Geometry check sheet. Reference: the model listing, model coordinates, mm. Coordinates: 2 decimals unless noted, no trailing zeros. Order: outer loops, then holes, each group sorted by start corner. A loop starts at its lowest first (then second) coordinate and runs counter-clockwise, first axis right, second up. Notation, with made-up numbers: (36, 7) -> (65, 7) arc R29 cw to (65, 30) -> close; hole circle Ø5 at (26.5, 11). An arc over 180 degrees is marked (long way). Answer in a Markdown table with one row per item. Add a question column.
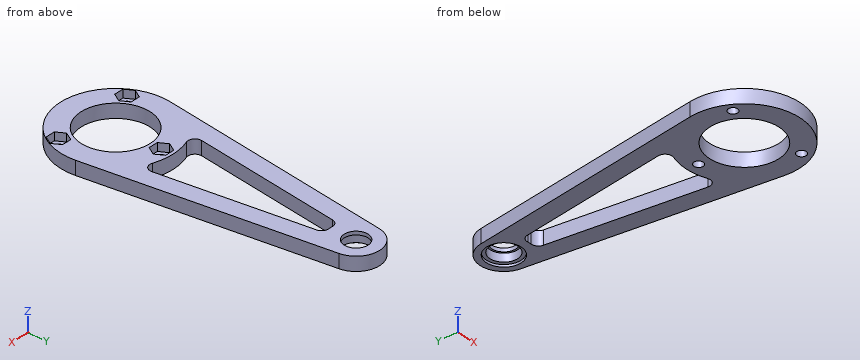
```python
from build123d import *

# Parameters (mm, degrees)
SKETCH_1_R          = 15
SKETCH_1_R_2        = 2
SKETCH_1_R_3        = 5.2
EXTRUDE_1_DEPTH     = 6
FILLET_1_R          = 3
CUT_EXTRUDE_1_DEPTH = 3.5
SKETCH_3_R          = 6
CUT_EXTRUDE_2_DEPTH = 4.5
SKETCH_4_R          = 7.5
CUT_EXTRUDE_3_DEPTH = 1


with BuildPart() as part:
    # 草图1 → 凸台-拉伸1 (new body)
    with BuildSketch(Plane.XY):
        with BuildLine():
            Line((-23.791815434, 3.154285714), (-10.111521559, 106.340571429))
            ThreePointArc((-10.111521559, 106.340571429), (0, 115.2), (10.111521559, 106.340571429))
            Line((10.111521559, 106.340571429), (23.791815434, 3.154285714))
            ThreePointArc((23.791815434, 3.154285714), (0, -24), (-23.791815434, 3.154285714))
        make_face()
        Circle(SKETCH_1_R, mode=Mode.SUBTRACT)
        with Locations((0, 20)):
            Circle(SKETCH_1_R_2, mode=Mode.SUBTRACT)
        with Locations((0, 105)):
            Circle(SKETCH_1_R_3, mode=Mode.SUBTRACT)
        with Locations((17.320508076, -10)):
            Circle(SKETCH_1_R_2, mode=Mode.SUBTRACT)
        with Locations((-17.320508076, -10)):
            Circle(SKETCH_1_R_2, mode=Mode.SUBTRACT)
        with BuildLine():
            Line((-13.336549876, 21.1456009), (-3.624239112, 94.402599807))
            ThreePointArc((-3.624239112, 94.402599807), (0, 93.8), (3.624239112, 94.402599807))
            Line((3.624239112, 94.402599807), (13.336549876, 21.1456009))
            ThreePointArc((13.336549876, 21.1456009), (0, 25), (-13.336549876, 21.1456009))
        make_face(mode=Mode.SUBTRACT)
    extrude(amount=EXTRUDE_1_DEPTH)

    # 圆角1
    fillet_1_edges = [part.edges().sort_by_distance(p)[0] for p in [
        (-13.336549876, 21.1456009, 3),
        (13.336549876, 21.1456009, 3),
        (3.624239112, 94.402599807, 3),
        (-3.624239112, 94.402599807, 3),
    ]]
    fillet(fillet_1_edges, radius=FILLET_1_R)

    # 草图2 → 切除-拉伸1 (cut)
    with BuildSketch(Plane.XY.offset(6)):
        Polygon((2.078460969, 16.4), (4.156921938, 20), (2.078460969, 23.6), (-2.078460969, 23.6), (-4.156921938, 20), (-2.078460969, 16.4), align=None)
        Polygon((19.398969045, -13.6), (21.477430014, -10), (19.398969045, -6.4), (15.242047107, -6.4), (13.163586138, -10), (15.242047107, -13.6), align=None)
        Polygon((-15.242047107, -13.6), (-13.163586138, -10), (-15.242047107, -6.4), (-19.398969045, -6.4), (-21.477430014, -10), (-19.398969045, -13.6), align=None)
    extrude(amount=-CUT_EXTRUDE_1_DEPTH, mode=Mode.SUBTRACT)

    # 草图3 → 切除-拉伸2 (cut)
    with BuildSketch(Plane(origin=(0, 0, 0), x_dir=(-1, 0, 0), z_dir=(0, 0, -1))):
        with Locations((0, 105)):
            Circle(SKETCH_3_R)
    extrude(amount=-CUT_EXTRUDE_2_DEPTH, mode=Mode.SUBTRACT)

    # 草图4 → 切除-拉伸3 (cut)
    with BuildSketch(Plane(origin=(0, 0, 0), x_dir=(-1, 0, 0), z_dir=(0, 0, -1))):
        with Locations((0, 105)):
            Circle(SKETCH_4_R)
    extrude(amount=-CUT_EXTRUDE_3_DEPTH, mode=Mode.SUBTRACT)


solid = part.part
```
(1) Cross-section at C-C (y = 70.5). Enter the section's corners in (x, z).
(2) Scan lines: line 1 along X through (y, z) = (-10, 1.9); line 2 along X through (y, z) = (35, 3.2); line 3 along X through (y, z) = (10, 1.95). Record each from-to range of solid material in increasing order.
(3) Go/stop test with flat-tipped pins: P1, Ø2, axis at x = -1, y = 21, coming from the +Z side; P2, Ø1.8, axis at x = -17, z = 4.5, coming from the -Y side; P3, Ø1.5, axis at x = 3.5, z = 2.5, coming from the +Y side. Record where each tip stops, or that it passes through.
(4) Cross-section at B-B (y = 105). Enter the section's corners in (x, z).
(5) Cross-section at A-A (y = 0). Enter the section's corners in (x, z).
Checks:
| question | item | result |
|---|---|---|
| 1 | outline | (-14.86, 0) -> (-6.79, 0) -> (-6.79, 6) -> (-14.86, 6) -> close; (6.79, 0) -> (14.86, 0) -> (14.86, 6) -> (6.79, 6) -> close |
| 2 | line 1 | -21.82 to -19.32, -15.32 to -11.18, 11.18 to 15.32, 19.32 to 21.82 |
| 2 | line 2 | -19.57 to -11.5, 11.5 to 19.57 |
| 2 | line 3 | -22.88 to -11.18, 11.18 to 22.88 |
| 3 | P1 | z = 2.5 |
| 3 | P2 | y = -17.8 |
| 3 | P3 | y = 114.82 |
| 4 | outline | (-10.29, 0) -> (-7.5, 0) -> (-7.5, 1) -> (-6, 1) -> (-6, 4.5) -> (-5.2, 4.5) -> (-5.2, 6) -> (-10.29, 6) -> close; (5.2, 4.5) -> (6, 4.5) -> (6, 1) -> (7.5, 1) -> (7.5, 0) -> (10.29, 0) -> (10.29, 6) -> (5.2, 6) -> close |
| 5 | outline | (-24, 0) -> (-15, 0) -> (-15, 6) -> (-24, 6) -> close; (15, 0) -> (24, 0) -> (24, 6) -> (15, 6) -> close |
